The drawing under review shows one solid part. Ordinate dimensions are in mm from its lowest x, y, z. A direction names the side the tool comes from. Round coordinates to 2 decimals unless told otherwise and drop trailing zeros. Write each loop counter-clockwise with the first axis right and the second up, starting at its lowest first coordinate (ties: lowest second). Pieces come first, ordered by that corner, then holes.
Item 1: Add section C-C (y = 22). Give the boundary of the cut face in (x, z), plus the area to 3 significant figures.
Item 2: Add section B-B (y = 7). Give the boundary of the cut face in (x, z).
Item 3: Clearance check with flat-ended pins moving along their axes: pin 1 Ø3 at (x, y) = (13, 18.5) entering from +Z; pin 2 Ø1 at (y, z) = (35.5, 9.5) entering from -X; pin 3 Ø1 at (x, z) = (8, 2.5) entering from +Y. State where each tip first meets the part, or that it passes through.
Item 4: To check wall thickness, follow L1, parallel to Y at x = 3, z = 8.25; L2, parallel to Z at x = 10, y = 23.5; L3, parallel to X at y = 29, z = 12.5. State the ranges of each line that lie inside material, in increasing order.
Item 5: Machinability: for the marked faces 1 and 2, which of the approach directions +Z, -Z, +X, -X, +Y, -Y give a long, thin tool a straight path to every point of the face, cutting with its end or side? Answer none if there is none.
Item 6: Add section A-A (x = 10). Give the boundary of the cut face in (y, z), plus the area to 3 significant figures.
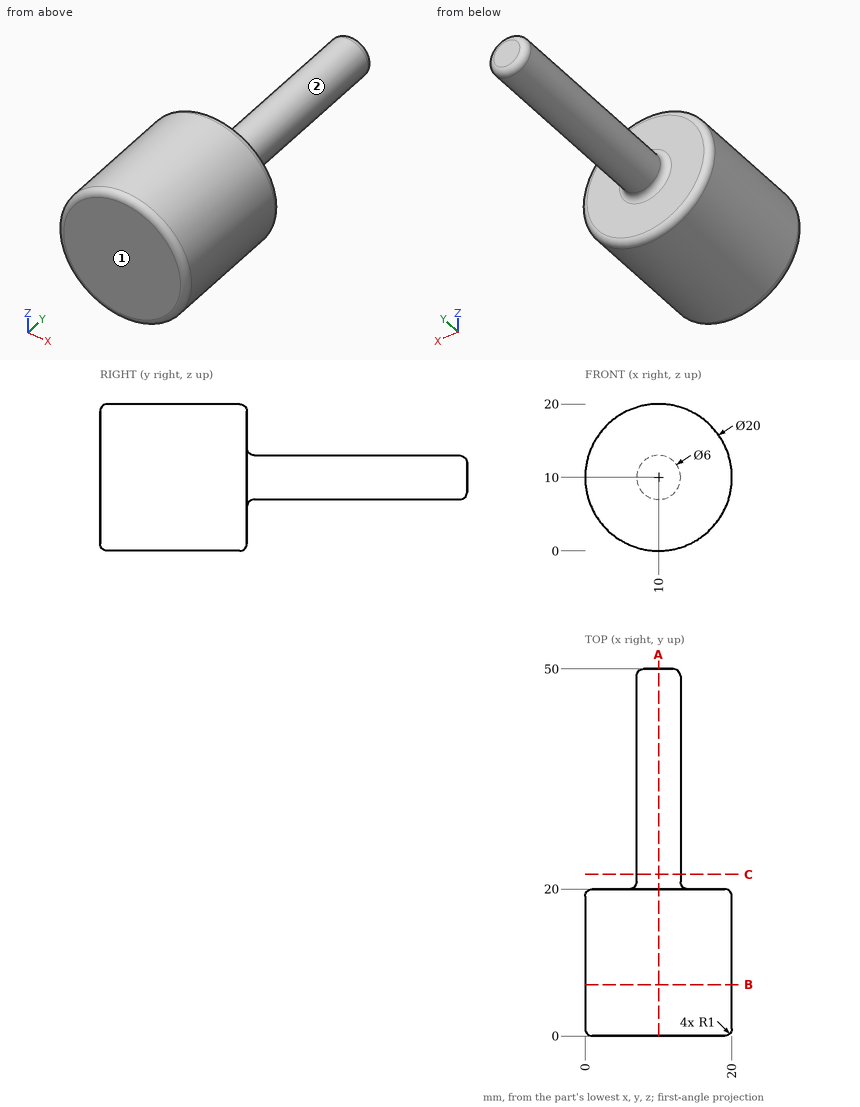
Numbers:
1. outline: circle Ø6 at (10, 10)
1. area: 28.3 mm2
2. outline: circle Ø20 at (10, 10)
3. pin 1: stops at z = 19.89
3. pin 2: stops at x = 7
3. pin 3: stops at y = 20
4. L1: y = 0 to 20
4. L2: z = 7 to 13
4. L3: x = 8.34 to 11.66
5. face 1: +Z, -Z, +X, -X, -Y
5. face 2: +Y
6. outline: (0, 1) arc R1 ccw to (1, 0) - (19, 0) arc R1 ccw to (20, 1) - (20, 6) arc R1 cw to (21, 7) - (49, 7) arc R1 ccw to (50, 8) - (50, 12) arc R1 ccw to (49, 13) - (21, 13) arc R1 cw to (20, 14) - (20, 19) arc R1 ccw to (19, 20) - (1, 20) arc R1 ccw to (0, 19) - close
6. area: 579 mm2
